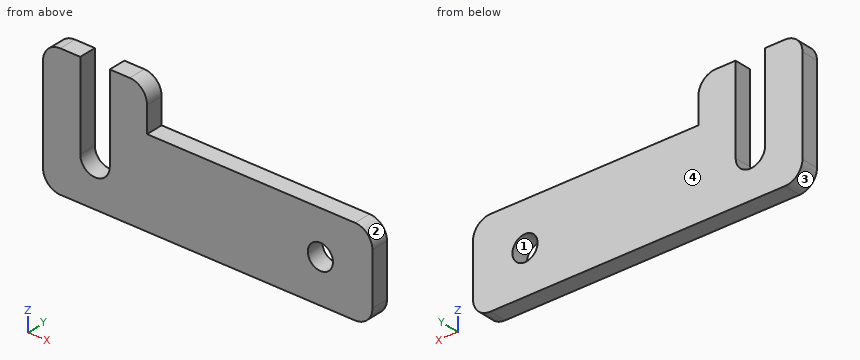
```python
from build123d import *

# Parameters (mm, degrees)
SKETCH_1_W             = 38
SKETCH_1_H             = 2
SM_BASE_FLANGE_1_DEPTH = 15
CUT_EXTRUDE_1_REACH    = 26.29
SKETCH_6_W             = 26
SKETCH_6_H             = 5
HOLE_WIZARD_M2_5_1_D   = 2.9
CUT_EXTRUDE_2_REACH    = 26.29
FILLET_1_R             = 2


# Sheet-metal steps are written as plain solids
with BuildPart() as part:
    # Sketch 1 → ﾍﾞｰｽ-ﾌﾗﾝｼﾞ1 (new body)
    with BuildSketch(Plane.XY):
        with Locations((0, -1)):
            Rectangle(SKETCH_1_W, SKETCH_1_H)
    extrude(amount=SM_BASE_FLANGE_1_DEPTH)

    # ｽｹｯﾁ6 → ｶｯﾄ - 押し出し1 (cut, up to next)
    with BuildSketch(Plane(origin=(0, 0, 0), x_dir=(1, 0, 0), z_dir=(0, 1, 0)), mode=Mode.PRIVATE) as cut_extrude_1_sk1:
        with Locations((6, -12.5)):
            Rectangle(SKETCH_6_W, SKETCH_6_H)
    cut_extrude_1_tool1 = extrude(cut_extrude_1_sk1.sketch, amount=-CUT_EXTRUDE_1_REACH, mode=Mode.PRIVATE) & part.part
    add(cut_extrude_1_tool1.solids().sort_by_distance((6, 0, 12.5))[0], mode=Mode.SUBTRACT)

    # M2.5 すきま穴1 (through all)
    with Locations(Plane(origin=(0, 0, 0), x_dir=(1, 0, 0), z_dir=(0, 1, 0))):
        with Locations((13, -5)):
            Hole(HOLE_WIZARD_M2_5_1_D / 2)

    # ｽｹｯﾁ9 → ｶｯﾄ - 押し出し2 (cut, up to next)
    with BuildSketch(Plane(origin=(0, 0, 0), x_dir=(1, 0, 0), z_dir=(0, 1, 0)), mode=Mode.PRIVATE) as cut_extrude_2_sk1:
        with BuildLine():
            Line((-11.3, -5), (-11.3, -15))
            ThreePointArc((-11.3, -15), (-13, -16.7), (-14.7, -15))
            Line((-14.7, -15), (-14.7, -5))
            ThreePointArc((-14.7, -5), (-13, -3.3), (-11.3, -5))
        make_face()
    cut_extrude_2_tool1 = extrude(cut_extrude_2_sk1.sketch, amount=-CUT_EXTRUDE_2_REACH, mode=Mode.PRIVATE) & part.part
    add(cut_extrude_2_tool1.solids().sort_by_distance((-13, 0, 10))[0], mode=Mode.SUBTRACT)

    # ﾌｨﾚｯﾄ1
    fillet_1_edges = [part.edges().sort_by_distance(p)[0] for p in [
        (-19, -1, 15),
        (19, -1, 10),
        (-7, -1, 15),
        (-19, -1, 0),
        (19, -1, 0),
    ]]
    fillet(fillet_1_edges, radius=FILLET_1_R)


solid = part.part
```
Can you work these out from the model? Positions are in its coordinate system, mm. Face numbers are marked on the shaded views. Give positions to 0.01 mm unless a question says otherwise; leave off trailing zeros. Loops run counter-clockwise (first coordinate to the right, second up) from the corner with the lowest first, then second, coordinate; pieces in that order, holes last. Notation, with made-up numbers: M 86.25,74.25 L 133.25,74.25 A18 cw 133.25,105.25 Z; hole C -33,80.5 d6. An arc over 180 degrees is marked long. Use one line per item in the form item = value. Start each with the question number.
(1) Please list where these lines run through material, in increasing order: line 1 (X direction, y = -1.4, z = 5); line 2 (Z direction, x = 13, y = -1.4); line 3 (X direction, y = -1.4, z = 5.75).
(2) Thinking about a two-plate mould opening in X: for the marked faces 1, 2, 3 and 4, which applies, released by +X, released by -X, zero draft, split by the parting line, or undercut?
(3) I want a section at B-B, the plane z = 7. Write out the boundary of the cut face in (x, y), and give its area (3 significant figures).
(4) I want a section at C-C, the plane y = -0.8. Write out the boundary of the cut face in (x, z), and give its area (3 significant figures).
(5) I want a section at A-A, the plane x = 13. Write out the boundary of the cut face in (y, z).
(6) I want a section at D-D, the plane x = -13. Write out the boundary of the cut face in (y, z), and give its area (3 significant figures).
(7) I'm going to push flat-ended pins straight in: P1, Ø1, axis at x = -2, z = 9.5, coming from the +Y side; P2, Ø0.6, axis at x = 3.5, y = -1, coming from the +Z side. Where does each tip first touch, or does it pass through?
Worked out:
q1.line_1 = -19 to -14.7, -11.3 to 11.55, 14.45 to 19
q1.line_2 = 0 to 3.55, 6.45 to 10
q1.line_3 = -19 to -14.7, -11.3 to 11.76, 14.24 to 19
q2.face_1 = undercut
q2.face_2 = released by +X
q2.face_3 = released by -X
q2.face_4 = zero draft
q3.outline = M -19,-2 L -14.7,-2 L -14.7,0 L -19,0 Z; M -11.3,-2 L 19,-2 L 19,0 L -11.3,0 Z
q3.area = 69.2 mm²
q4.outline = M -19,2 A2 ccw -17,0 L 17,0 A2 ccw 19,2 L 19,8 A2 ccw 17,10 L -7,10 L -7,13 A2 ccw -9,15 L -11.3,15 L -11.3,5 A1.7 cw -14.7,5 L -14.7,15 L -17,15 A2 ccw -19,13 Z; hole C 13,5 d2.9
q4.area = 391 mm²
q5.outline = M -2,0 L 0,0 L 0,3.55 L -2,3.55 Z; M -2,6.45 L 0,6.45 L 0,10 L -2,10 Z
q6.outline = M -2,0 L 0,0 L 0,3.3 L -2,3.3 Z
q6.area = 6.60 mm²
q7.P1 = 0
q7.P2 = 10
